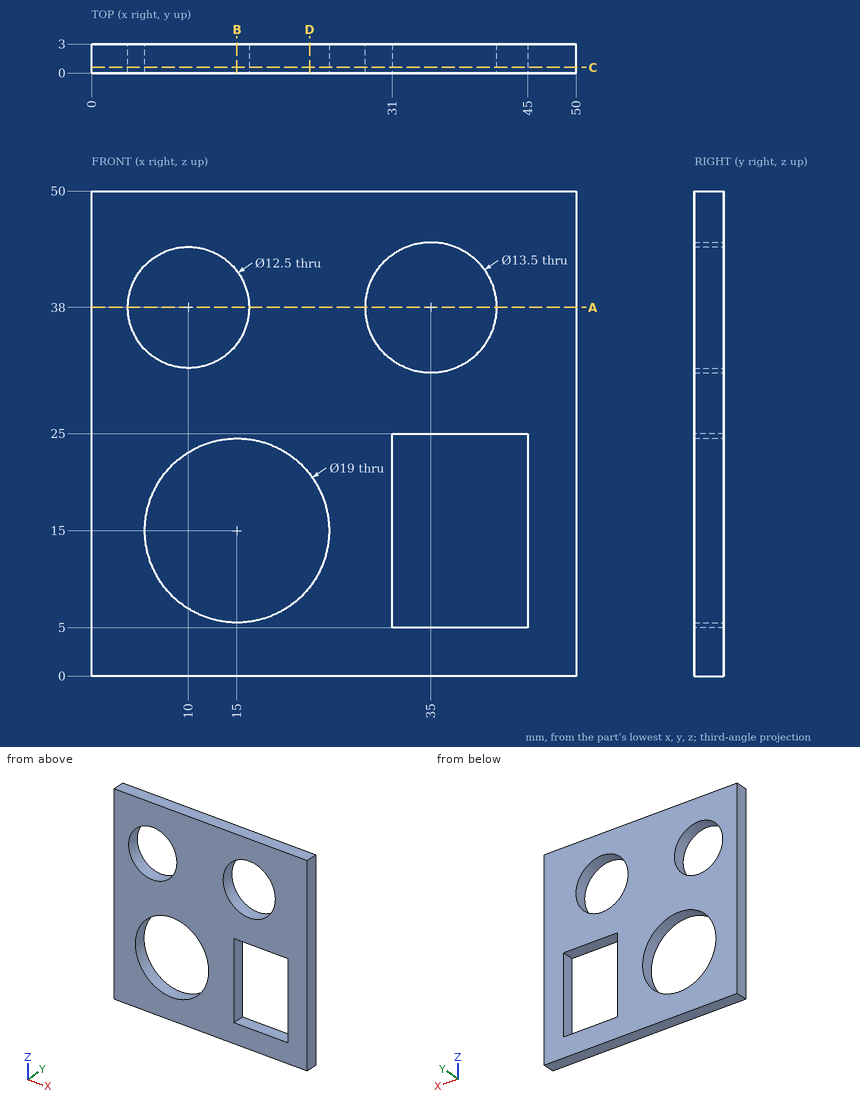
Study the drawing (mm; zero at the part's minimum x, y, z) and answer. Round coordinates to 2 decimals unless told otherwise and drop trailing zeros. Order: outer loops, then holes, each group sorted by start corner. A loop starts at its lowest first (then second) coordinate and runs counter-clockwise, first axis right, second up. Notation, with made-up numbers: M -26.5,11.25 L 7.5,11.25 A23 cw 7.5,43.25 Z; hole C 25.25,13 d2. An arc over 180 degrees is marked long. One line per item, written item: value.
Q1. Find section B-B on x = 15. Write down the section's boundary in (y, z).
Derived:
outline: M 0,0 L 3,0 L 3,5.5 L 0,5.5 Z; M 0,24.5 L 3,24.5 L 3,34.25 L 0,34.25 Z; M 0,41.75 L 3,41.75 L 3,50 L 0,50 Z
Q2. Find section A-A on z = 38. Write down the section's boundary in (x, y).
Derived:
outline: M 0,0 L 3.75,0 L 3.75,3 L 0,3 Z; M 16.25,0 L 28.25,0 L 28.25,3 L 16.25,3 Z; M 41.75,0 L 50,0 L 50,3 L 41.75,3 Z
Q3. Find section C-C on y = 0.6. Write down the section's boundary in (x, z).
Derived:
outline: M 0,0 L 50,0 L 50,50 L 0,50 Z; hole C 10,38 d12.5; hole C 15,15 d19; hole C 35,38 d13.5; hole M 31,5 L 45,5 L 45,25 L 31,25 Z
Q4. A flat-ended cylindrical pin translates along its axis: pin 1 (2 mm diameter, centred on x = 36, z = 23.5, fed in from +Y). Find the tip coordinate at first contact, or state that the pin passes through.
Derived:
pin 1: through
Q5. Find section D-D on x = 22.5. Write down the section's boundary in (y, z), then the cut area to 3 significant figures.
Derived:
outline: M 0,0 L 3,0 L 3,9.17 L 0,9.17 Z; M 0,20.83 L 3,20.83 L 3,50 L 0,50 Z
area: 115 mm²
Q6. Straight lines are drawn through the part: line 1 (X direction, y = 2.4, z = 38); line 2 (X direction, y = 1.2, z = 15); line 3 (Z direction, x = 32, y = 1.5). For each, find the intervals that lie inside material, in ascending order.
Derived:
line 1: 0 to 3.75, 16.25 to 28.25, 41.75 to 50
line 2: 0 to 5.5, 24.5 to 31, 45 to 50
line 3: 0 to 5, 25 to 31.95, 44.05 to 50
